Here's how the part is built. I have some questions about the finished solid (model axes, mm). Face numbers are marked on the shaded views. Coordinates: 2 decimals unless noted, no trailing zeros. Write each loop counter-clockwise with the first axis right and the second up, starting at its lowest first coordinate (ties: lowest second). Pieces come first, ordered by that corner, then holes.
(1) Please list where these lines run through material, in increasing order: probe 1 along Y at (x, z) = (-1, 6.75); probe 2 along Y at (x, z) = (27.5, 8.75); probe 3 along X at (y, z) = (-3, 7).
(2) For pin 1 Ø2 at (y, z) = (-42, 7) entering from +X; pin 2 Ø4 at (y, z) = (29, 7.5) entering from -X; pin 3 Ø8 at (x, y) = (0, 0) entering from -Z; pin 4 Ø6 at (x, z) = (4, 4) entering from -Y, each with a flat end and sliding along its axis, tell me the tip position at first contact or that it passes through.
(3) Thinking about a two-plate mould opening in Y: for the marked faces 1, 2 and 3, which applies, released by +Y, released by -Y, zero draft, split by the parting line, or undercut?
(4) Imagine slicing it at C-C, the plane y = 0. List the corners of the cut face in (x, z) for me, plus the area to 3 significant figures.
(5) Imagine slicing it at A-A, the plane x = 27. List the corners of the cut face in (y, z) for me.
(6) Imagine slicing it at B-B, the plane x = 0. List the corners of the cut face in (y, z) for me.
(7) Imagine slicing it at D-D, the plane z = 7. List the corners of the cut face in (x, y) for me.
Autodesk Inventor part; units mm, degrees
ref_plane "YZ Plane" through (0, 0, 0) normal (1, 0, 0) x (0, 1, 0)
ref_plane "XZ Plane" through (0, 0, 0) normal (0, 1, 0) x (-1, 0, 0)
ref_plane "XY Plane" through (0, 0, 0) normal (0, 0, 1) x (1, 0, 0)
sketch "Sketch1" plane through (0, 0, 0) normal (0, 0, 1) x (1, 0, 0)
  circle A0 centre (0, 0) radius 4.5
  line L0 (0, 0) -> (27.3538, 43.7752) construction
  line L1 (0, -76.1552) -> (0, 69.6997) construction
  line L2 (0, 0) -> (0, -51.6188) construction
  circle A1 centre (0, -51.6188) radius 1.7
  circle A2 centre (27.3538, 43.7752) radius 1.7
  arc A3 (30.6767, 42.1478) -> (24.4345, 46.0484) centre (27.3538, 43.7752) ccw
  arc A4 (-3.6804, -51.9996) -> (3.6804, -51.9996) centre (0, -51.6188) ccw
  line L3 (0, 0) -> (7.9488, 12.7207) construction
  circle A5 centre (7.9488, 12.7207) radius 2
  line L4 (0, 0) -> (0, -15) construction
  circle A6 centre (0, -15) radius 2
  line L5 (-7.1107, 5.5369) -> (24.4345, 46.0484)
  line L6 (-8.9644, -0.9275) -> (-3.6804, -51.9996)
  line L7 (8.7873, -2.6385) -> (30.6767, 42.1478)
  line L8 (8.7873, -2.6385) -> (3.6804, -51.9996)
  arc A7 (-7.1107, 5.5369) -> (-8.9644, -0.9275) centre (0, 0) ccw
  point P0 (8.0937, -3.9639)
  dimension "d0" = 9
  dimension "d2" = 32
  dimension "d3" = 51.6188
  dimension "d4" = 51.6188
  dimension "d5" = 3.4
  dimension "d6" = 3.4
  dimension "d7" = 3.7
  dimension "d8" = 3.7
  dimension "d9" = 15
  dimension "d10" = 4
  dimension "d11" = 15
  dimension "d12" = 4
extrude "Extrusion1" add sketch "Sketch1" along normal blind 10
equation "\"d3\" = d4"
properties part number "Lever" material "Steel"
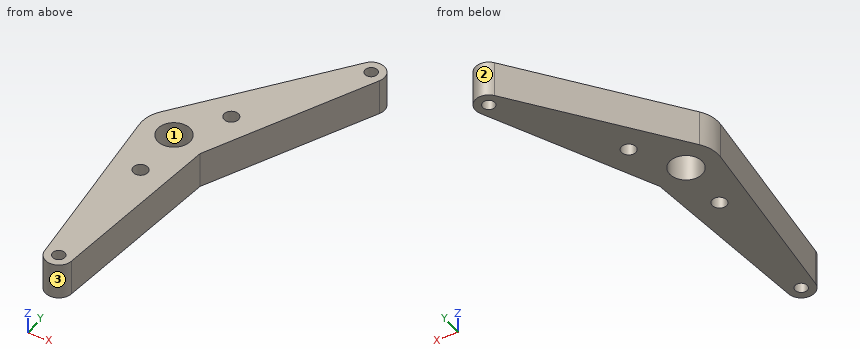
Recorded:
1. probe 1: y = -55.18 to -52.99, -50.24 to -16.73, -13.27 to -4.39, 4.39 to 13.38
1. probe 2: y = 35.65 to 42.08, 45.47 to 47.47
1. probe 3: x = -8.75 to -3.35, 3.35 to 8.75
2. pin 1: stops at x = 4.82
2. pin 2: stops at x = 9.6
2. pin 3: passes through
2. pin 4: stops at y = -55.18
3. face 1: undercut
3. face 2: split by the parting line
3. face 3: released by -Y
4. outline: (-9.01, 0) - (-4.5, 0) - (-4.5, 10) - (-9.01, 10) - close; (4.5, 0) - (10.08, 0) - (10.08, 10) - (4.5, 10) - close
4. area: 101 mm2
5. outline: (34.63, 0) - (42.11, 0) - (42.11, 10) - (34.63, 10) - close; (45.44, 0) - (47.46, 0) - (47.46, 10) - (45.44, 10) - close
6. outline: (-55.32, 0) - (-53.32, 0) - (-53.32, 10) - (-55.32, 10) - close; (-49.92, 0) - (-17, 0) - (-17, 10) - (-49.92, 10) - close; (-13, 0) - (-4.5, 0) - (-4.5, 10) - (-13, 10) - close; (4.5, 0) - (14.67, 0) - (14.67, 10) - (4.5, 10) - close
7. outline: (-8.96, -0.93) - (-3.68, -52) arc R3.7 ccw to (3.68, -52) - (8.79, -2.64) - (30.68, 42.15) arc R3.7 ccw to (24.43, 46.05) - (-7.11, 5.54) arc R9.01 ccw to start; hole circle Ø9 at (0, 0); hole circle Ø4 at (0, -15); hole circle Ø3.4 at (0, -51.62); hole circle Ø4 at (7.95, 12.72); hole circle Ø3.4 at (27.35, 43.78)
